Input: part model. Units: mm. Frame: model coordinates. Coordinates: 2 decimals unless noted, no trailing zeros. Loops run counter-clockwise (first coordinate to the right, second up) from the corner with the lowest first, then second, coordinate; pieces in that order, holes last.
Item 1: Ray query, line 1 along Z through (x, y) = (0, 71); line 2 along X through (y, z) = (62, 15.24); line 3 along X through (y, z) = (27.5, 31.5). Return the intervals inside material, ascending.
Item 2: Section B-B on z = 0. Return loops of the section in (x, y).
Item 3: Contact query for flat-ended pins moving along their axis: P1, Ø3, axis at x = 19, y = 22, coming from the +Z side; P2, Ø1, axis at x = 3, y = 42.5, coming from the -Z side; P3, Ø6, axis at y = 29, z = -7.5, coming from the -X side; P4, Ø1, axis at x = 19.5, y = 47.5, coming from the +Z side. Output: stop coordinate, or through.
Item 4: Section A-A on x = -10. Return loops of the section in (y, z).
Item 5: Section D-D on x = 0. Return loops of the section in (y, z).
Item 6: Section C-C on z = 17.5. Return loops of the section in (x, y).
```python
from build123d import *

# Parameters (mm, degrees)
F0_W     = 55.88
F0_H     = 30.48
F1_DEPTH = 127
F2_R     = 21.4884
F3_DEPTH = 127.001
F5_DEPTH = 55.881


with BuildPart() as f1:
    # F0 (on Front) → F1 (new body)
    with BuildSketch(Plane.XZ):
        with BuildLine():
            Line((-27.94, 15.24), (27.94, 15.24))
            ThreePointArc((27.94, 15.24), (0, 43.18), (-27.94, 15.24))
        make_face()
        Rectangle(F0_W, F0_H)
    extrude(amount=-F1_DEPTH)

    # F2 (on face) → F3 (cut, through all)
    with BuildSketch(Plane.XZ):
        with Locations((0, 15.24)):
            Circle(F2_R)
    extrude(amount=-F3_DEPTH, mode=Mode.SUBTRACT)

    # F4 (on face) → F5 (cut, through all)
    with BuildSketch(Plane.YZ.offset(27.94)):
        Polygon((267.642255, 109.563633), (0, -15.24), (267.642255, -15.24), align=None)
    extrude(amount=-F5_DEPTH, mode=Mode.SUBTRACT)


solid = f1.part
```
Results found:
1. line 1: z = 36.73 to 43.18
1. line 2: x = -27.94 to -21.49, 21.49 to 27.94
1. line 3: x = -22.72 to -14.05, 14.05 to 22.72
2. outline: (-27.94, 0) - (-15.15, 0) - (-15.15, 32.68) - (-27.94, 32.68) - close; (15.15, 0) - (27.94, 0) - (27.94, 32.68) - (15.15, 32.68) - close
3. P1: stops at z = 37.02
3. P2: stops at z = 36.44
3. P3: passes through
3. P4: stops at z = 35.73
4. outline: (0, -15.24) - (24.58, -3.78) - (0, -3.78) - close; (0, 34.26) - (106.15, 34.26) - (121.31, 41.33) - (0, 41.33) - close
5. outline: (0, -15.24) - (19.28, -6.25) - (0, -6.25) - close; (0, 36.73) - (111.45, 36.73) - (125.28, 43.18) - (0, 43.18) - close
6. outline: (-27.85, 0) - (-21.37, 0) - (-21.37, 70.21) - (-27.85, 70.21) - close; (21.37, 0) - (27.85, 0) - (27.85, 70.21) - (21.37, 70.21) - close
